Input: part model. Units: mm. Frame: model coordinates. Give positions to 0.01 mm unless a question says otherwise; leave off trailing zeros. Write each loop counter-clockwise with the first axis right and the second up, starting at its lowest first coordinate (ties: lowest second). Pieces come first, ordered by that corner, then holes. Notation, with made-up numbers: (41, 32.25) -> (97, 32.25) arc R22 cw to (97, 59.25) -> close; hole circle Ø1 at (31.25, -32.75). An arc over 180 degrees is marked (long way). Return JSON: item names as keys, results as strings. Group by question number.
Item 1: Section B-B, the plane x = 174.5. Return loops of the section in (y, z).
Item 2: Section A-A, the plane z = -4. Return loops of the section in (x, y).
Item 3: Line query: line 1 (X direction, y = 0.9, z = -4); line 2 (Z direction, x = -94.5, y = 1.5); line 3 (Z direction, x = 181, y = 4.25). Output: solid intervals per line, ascending. Write a range as [from, to].
Item 4: Section C-C, the plane x = 27.5. Return loops of the section in (y, z).
Item 5: Pin query (flat end, axial travel): P1, Ø3.5, axis at x = 47.5, y = 3, coming from the -Z side; P2, Ø0.6, axis at y = 0.5, z = -3.5, coming from the +X side; P3, Ø7, axis at x = 39.5, z = 20, coming from the +Y side; P4, Ø1.5, axis at y = 4.25, z = 6.75, coming from the +X side. Return the tip coordinate at first contact, or that it passes through.
Autodesk Fusion 360 part; units mm, degrees
sketch "base" plane through (0, 0, 0) normal (0, 1, 0) x (1, 0, 0)
  line L0 (-100, 1.5) -> (180, 1.5)
  line L1 (180, 1.5) -> (180, -13.5)
  line L2 (180, -13.5) -> (-100, -13.5)
  line L3 (-100, -13.5) -> (-100, 1.5)
  line L4 (-100, -13.5) -> (180, -13.5)
  line L5 (180, -13.5) -> (180, -17.5)
  line L6 (180, -17.5) -> (-100, -17.5)
  line L7 (-100, -17.5) -> (-100, -13.5)
  line L8 (-100, 1.5) -> (-85, 1.5) construction
  circle A0 centre (-94.5, 4) radius 2.5
  line L9 (-100, 1.5) -> (-100, 7.5)
  line L10 (-100, 7.5) -> (-98, 9.5)
  line L11 (-85, 1.5) -> (-85, 7.5)
  line L12 (-85, 7.5) -> (-87, 9.5)
  line L13 (-87, 9.5) -> (-98, 9.5)
  line L14 (40, 6.0385) -> (40, -33.3841) construction
  line L15 (167, 9.5) -> (178, 9.5)
  line L16 (180, 7.5) -> (178, 9.5)
  line L17 (180, 1.5) -> (180, 7.5)
  circle A1 centre (174.5, 4) radius 2.5
  line L18 (165, 7.5) -> (167, 9.5)
  line L19 (165, 1.5) -> (165, 7.5)
  circle A2 centre (40, -18.5) radius 2.5
  line L20 (34.5, -21.5) -> (36.5, -21.5) construction
  line L21 (36.5, -21.5) -> (36.5, -23.5) construction
  line L22 (34.5, -21.5) -> (36.5, -23.5)
  line L23 (36.5, -23.5) -> (40, -23.5)
  circle A3 centre (40, -18.5) radius 3.75 construction
  circle A4 centre (40, -18.5) radius 4
  line L24 (34.5, -21.5) -> (34.5, -17.5)
  line L25 (45.5, -21.5) -> (45.5, -17.5)
  line L26 (45.5, -21.5) -> (43.5, -23.5)
  line L27 (43.5, -23.5) -> (40, -23.5)
  line L28 (-98, -13) -> (-98, -1) construction
  line L29 (-98, -1) -> (-104, -1)
  line L30 (-104, -1) -> (-104, -13.5)
  line L31 (-104, -13.5) -> (-100, -17.5)
  line L32 (-98, -1) -> (-98, -13.5)
  line L33 (178, -13) -> (178, -1) construction
  line L34 (178, -1) -> (178, -13.5)
  line L35 (178, -1) -> (184, -1)
  line L36 (184, -1) -> (184, -13.5)
  line L37 (184, -13.5) -> (180, -17.5)
  circle A5 centre (-94.5, 4) radius 3.75 construction
  circle A6 centre (174.5, 4) radius 3.75 construction
  dimension "d1" = 280
  dimension "d2" = 15
  dimension "d3" = 4
  dimension "d4" = 280
  dimension "d5" = 15
  dimension "d7" = 5
  dimension "d8" = 2.5
  dimension "d11" = 140
  dimension "d16" = 5
  dimension "d17" = 5
  dimension "d20" = 2
  dimension "d21" = 2
  dimension "d22" = 7.5
  dimension "d23" = 8
  dimension "d29" = 12.5
  dimension "d42" = 7.5
  dimension "d43" = 7.5
extrude "Extrude1" add sketch "base" along normal blind 2 contours L0 L1 L2 L3 L4 L29 L32 L34 L35 | L0 L9 L10 L11 L12 L13 | L0 L15 L16 L17 L18 L19 | L2 L3 L4 L29 L32 | L1 L2 L4 L34 L35 | L6 L22 L23 A4 L24 L25 L26 L27 | L6 A2 A4 | L6 A2 A4 makes body 1 at (-1.6667, 0, 8.5) makes body 2 at (39.9377, 0, 22.6643)
extrude "Extrude2" add sketch "base" along normal blind 5 contours L2 L4 L5 L6 L7 A4 bodies 1 2
chamfer "Chamfer1" distance 2 angle 45 2 edges at (-31.9365, 5, 17.5) (111.9365, 5, 17.5) on bodies 1
extrude "Extrude3" add sketch "base" along normal blind 6.5 contours L2 L3 L4 L29 L32 | L3 L7 L29 L30 L31 | L1 L5 L35 L36 L37 | L1 L2 L4 L34 L35 bodies 1
chamfer "Chamfer2" distance 2 angle 45 4 edges at (182, 6.5, 15.5) (184, 6.5, 7.25) (-102, 6.5, 15.5) (-104, 6.5, 7.25) on bodies 1
sketch "Sketch2" plane through (-104, 0, 0) normal (-1, 0, 0) x (0, 0, 1)
  line L0 (13.5, 4.5) -> (1, 4.5)
  line L1 (1, 4.5) -> (1, 0)
  line L2 (1, 0) -> (13.5, 0)
  line L3 (13.5, 0) -> (13.5, 4.5)
  circle A0 centre (3.2461, 4.25) radius 1.25
  line L4 (-7.5, 2) -> (1, 2)
  circle A1 centre (3.2461, 4.25) radius 1.25
  circle A2 centre (6.7461, 4.25) radius 1.25
  circle A3 centre (10.2461, 4.25) radius 1.25
  dimension "d33" = 2.5
  dimension "d36" = 2.25
  dimension "d37" = 2.5
  dimension "d38" = 2.5
  dimension "d39" = 2.5
extrude "Extrude4" cut sketch "Sketch2" against normal blind 300 contours L0 A3 | L0 A3 | L0 A2 | L0 A2 | L0 A0 A1 | L0 A0 A1 bodies 1
chamfer "Chamfer4" distance 2 angle 45 2 edges at (180, 5.75, 13.5) (-100, 5.75, 13.5) on bodies 1
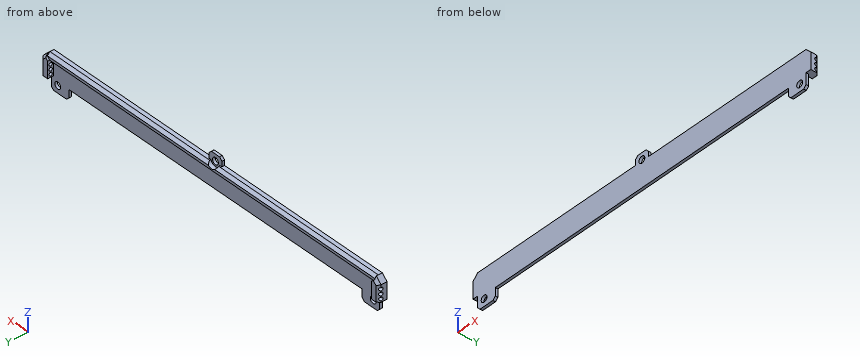
Answer below:
{
 "1": {"outline": "(0, -9.5) -> (2, -9.5) -> (2, -6.5) -> (0, -6.5) -> close; (0, -1.5) -> (2, -1.5) -> (2, 13.5) -> (5, 13.5) -> (5, 15.5) -> (3, 17.5) -> (0, 17.5) -> close"},
 "2": {"outline": "(-100, 0) -> (-97, 0) -> (-97, 2) -> (-100, 2) -> close; (-92, 0) -> (-85, 0) -> (-85, 2) -> (-92, 2) -> close; (165, 0) -> (172, 0) -> (172, 2) -> (165, 2) -> close; (177, 0) -> (180, 0) -> (180, 2) -> (177, 2) -> close"},
 "3": {"line 1": "x = [-100, -97], [-92, -85], [165, 172], [177, 180]", "line 2": "z = [-9.5, -6.5], [-1.5, 17.5]", "line 3": "z = [1, 2], [4.5, 5.5], [8, 9], [11.5, 16.5]"},
 "4": {"outline": "(0, -1.5) -> (2, -1.5) -> (2, 13.5) -> (5, 13.5) -> (5, 15.5) -> (3, 17.5) -> (0, 17.5) -> close"},
 "5": {"P1": "stops at z = -1.5", "P2": "stops at x = 180", "P3": "stops at y = 2", "P4": "passes through"}
}
